Geometry: final body of the model. Coordinates: model frame, mm. Coordinates: 2 decimals unless noted, no trailing zeros. Order: outer loops, then holes, each group sorted by start corner. A loop starts at its lowest first (then second) coordinate and runs counter-clockwise, first axis right, second up. Notation, with made-up numbers: M 52.5,-27 L 86.5,-27 A32 ccw 86.5,3 Z; hole C 6,50.25 d9. An arc over 180 degrees is marked long. One line per question, with ' | ' between items.
from build123d import *

# Parameters (mm, degrees)
SKETCH_R        = 36.2
SKETCH_R_2      = 32.65
PAD_DEPTH       = 5
CHAMFER_SIZE    = 1
CHAMFER001_SIZE = 0.3


with BuildPart() as part:
    # Sketch → Pad (new body)
    with BuildSketch(Plane.XY):
        Circle(SKETCH_R)
        Circle(SKETCH_R_2, mode=Mode.SUBTRACT)
    extrude(amount=PAD_DEPTH)

    # Chamfer
    chamfer_edges = [part.edges().sort_by_distance(p)[0] for p in [
        (-32.65, 0, 5),
    ]]
    chamfer(chamfer_edges, length=CHAMFER_SIZE)

    # Chamfer001
    chamfer001_edges = [part.edges().sort_by_distance(p)[0] for p in [
        (-36.2, 0, 0),
        (-32.65, 0, 0),
    ]]
    chamfer(chamfer001_edges, length=CHAMFER001_SIZE)


solid = part.part
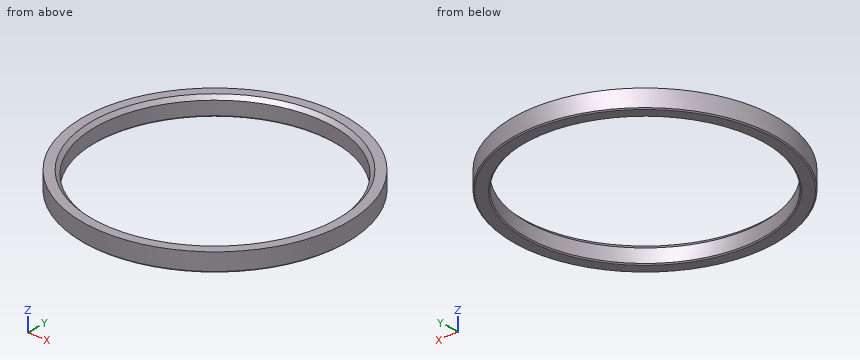
1. Section A-A, the plane y = 0. Output: boundary loops of the cut face in (x, z), and give its area (3 significant figures).
Response values:
outline: M -36.2,0.3 L -35.9,0 L -32.95,0 L -32.65,0.3 L -32.65,4 L -33.65,5 L -36.2,5 Z; M 32.65,0.3 L 32.95,0 L 35.9,0 L 36.2,0.3 L 36.2,5 L 33.65,5 L 32.65,4 Z | area: 34.3 mm^2
2. Material intervals for line 1 (Y direction, x = 0, z = 2.35); line 2 (X direction, y = -8.5, z = 2.9); line 3 (X direction, y = 12, z = 4.35), sorted ascending. Write a range as [from, to].
Response values:
line 1: y = [-36.2, -32.65], [32.65, 36.2] | line 2: x = [-35.19, -31.52], [31.52, 35.19] | line 3: x = [-34.15, -30.74], [30.74, 34.15]
3. Pin query (flat end, axial travel): P1, Ø1.5, axis at x = -15.5, z = 3.5, coming from the -Y side; P2, Ø2, axis at x = 12, y = 28.5, coming from the +Z side; P3, Ø1.5, axis at x = -11.5, z = 3.5, coming from the -Y side; P4, Ø1, axis at y = -9.5, z = 1.5, coming from the -X side. Return the tip coordinate at first contact, or that it passes through.
Response values:
P1: stops at y = -33.06 | P2: passes through | P3: stops at y = -34.57 | P4: stops at x = -35.06
4. Section C-C, the plane z = 3.2. Output: boundary loops of the cut face in (x, y).
Response values:
outline: C 0,0 d72.4; hole C 0,0 d65.3
